from build123d import *

# Parameters (mm, degrees)
SKETCH1_R           = 2
SKETCH1_R_2         = 1.5
SKETCH1_W           = 41
SKETCH1_H           = 20
BOSS_EXTRUDE1_DEPTH = 10


with BuildPart() as part:
    # Sketch1 → Boss-Extrude1 (new body)
    with BuildSketch(Plane.XY):
        with BuildLine():
            Line((-15.536480687, 29.570815451), (44.463519313, 29.570815451))
            ThreePointArc((44.463519313, 29.570815451), (51.534587125, 26.641883263), (54.463519313, 19.570815451))
            Line((54.463519313, 19.570815451), (54.463519313, -15.429184549))
            Line((54.463519313, -15.429184549), (-25.536480687, -15.429184549))
            Line((-25.536480687, -15.429184549), (-25.536480687, 19.570815451))
            ThreePointArc((-25.536480687, 19.570815451), (-22.607548499, 26.641883263), (-15.536480687, 29.570815451))
        make_face()
        with Locations((-10.036480687, 20.570815451)):
            Circle(SKETCH1_R, mode=Mode.SUBTRACT)
        with Locations((38.963519313, 8.570815451)):
            Circle(SKETCH1_R, mode=Mode.SUBTRACT)
        with Locations(Location((-10.036480687, 8.570815451, 0), (0, 0, 180))):
            Circle(SKETCH1_R, mode=Mode.SUBTRACT)
        with Locations(Location((38.963519313, 20.570815451, 0), (0, 0, 180))):
            Circle(SKETCH1_R, mode=Mode.SUBTRACT)
        with Locations((-19.536480687, -0.429184549)):
            Circle(SKETCH1_R_2, mode=Mode.SUBTRACT)
        with Locations((-19.536480687, 9.570815451)):
            Circle(SKETCH1_R_2, mode=Mode.SUBTRACT)
        with Locations(Location((48.463519313, 9.570815451, 0), (0, 0, 180))):
            Circle(SKETCH1_R_2, mode=Mode.SUBTRACT)
        with Locations(Location((48.463519313, -0.429184549, 0), (0, 0, 180))):
            Circle(SKETCH1_R_2, mode=Mode.SUBTRACT)
        with Locations((14.463519313, 14.570815451)):
            Rectangle(SKETCH1_W, SKETCH1_H, mode=Mode.SUBTRACT)
    extrude(amount=BOSS_EXTRUDE1_DEPTH)


solid = part.part
Geometry: final body of the model. Coordinates: model frame, mm. A direction names the side the tool comes from. Give positions to 0.01 mm unless a question says otherwise; leave off trailing zeros. Write each loop counter-clockwise with the first axis right and the second up, starting at its lowest first coordinate (ties: lowest second). Pieces come first, ordered by that corner, then holes. Notation, with made-up numbers: (86, 81.25) - (91, 81.25) arc R12 cw to (91, 101.25) - close; hole circle Ø5 at (-29, -27.5). An arc over 180 degrees is marked (long way). Return JSON: item names as keys, results as strings. Group by question number.
1) Line query: line 1 (Y direction, x = 31, z = 6.5); line 2 (X direction, y = -1, z = 6.5); line 3 (X direction, y = 6, z = 7.25). Output: solid intervals per line, ascending.
2) Set-up query: faces 4 (the flat face through (-25.536, 2, 5)), 5 (the flat face through (14, 4.571, 5)). Return all of +Z, -Z, +X, -X, +Y, -Y with unobstructed straight access to the full face (end or side cutting, diameter ignored); none if empty.
3) Section C-C on z = 1.25. State how many separate pieces and enclosed holes the cut face has, plus the area to 3 significant figures.
4) Mould query, pull axis Y, two halves, no side actions, for faces 1 (the flat face through (34.964, 14, 5)), 2 (the flat face through (15, 2, 0)), 3 (the cylindrical face through (-22.685, 26.564, 4.93)). Classes: released by +Y, released by -Y, zero draft, split by the parting line, or undercut.
5) Section B-B on y = 14. Return the cut outline in (x, z).
6) Section A-A on x = 29. Return the cut outline in (y, z), plus the area to 3 significant figures.
Filled in:
{
 "1": {"line 1": "y = -15.43 to 4.57, 24.57 to 29.57", "line 2": "x = -25.54 to -20.92, -18.15 to 47.08, 49.85 to 54.46", "line 3": "x = -25.54 to -6.04, 34.96 to 54.46"},
 "2": {"face 4": "+Z, -Z, -X, +Y, -Y", "face 5": "+Z, -Z"},
 "3": {"separate pieces": "1", "enclosed holes": "9", "area": "2,660 mm^2"},
 "4": {"face 1": "undercut", "face 2": "zero draft", "face 3": "released by +Y"},
 "5": {"outline": "(-25.54, 0) - (-6.04, 0) - (-6.04, 10) - (-25.54, 10) - close; (34.96, 0) - (54.46, 0) - (54.46, 10) - (34.96, 10) - close"},
 "6": {"outline": "(-15.43, 0) - (4.57, 0) - (4.57, 10) - (-15.43, 10) - close; (24.57, 0) - (29.57, 0) - (29.57, 10) - (24.57, 10) - close", "area": "250 mm^2"}
}
